```python
from build123d import *

# Parameters (mm, degrees)
SKETCH1_W           = 92.6
SKETCH1_H           = 300
BOSS_EXTRUDE1_DEPTH = 3
SKETCH3_R           = 2.25
SKETCH3_W           = 8.48
SKETCH3_H           = 51.5
SKETCH3_H_2         = 50
SKETCH3_W_2         = 5
SKETCH3_H_3         = 53
CUT_EXTRUDE2_DEPTH  = 10
FILLET1_R           = 2
SKETCH4_R           = 1.85
CUT_EXTRUDE3_DEPTH  = 5
SKETCH5_R           = 1.85
CUT_EXTRUDE4_DEPTH  = 10
SKETCH6_R           = 1.85
CUT_EXTRUDE5_DEPTH  = 8.5
CUT_EXTRUDE6_DEPTH  = 8.5
SKETCH9_R           = 1.85
CUT_EXTRUDE7_DEPTH  = 10


with BuildPart() as part:
    # Sketch1 → Boss-Extrude1 (new body)
    with BuildSketch(Plane.XY):
        Rectangle(SKETCH1_W, SKETCH1_H)
    extrude(amount=BOSS_EXTRUDE1_DEPTH)

    # Sketch3 → Cut-Extrude2 (cut)
    with BuildSketch(Plane.XY):
        with Locations((-42.06, 75)):
            Circle(SKETCH3_R)
        with Locations((42.06, 125)):
            Circle(SKETCH3_R)
        with Locations((42.06, 25)):
            Circle(SKETCH3_R)
        with Locations((42.06, -75)):
            Circle(SKETCH3_R)
        with Locations((-42.06, -25)):
            Circle(SKETCH3_R)
        with Locations((-42.06, -125)):
            Circle(SKETCH3_R)
        with Locations((-42.06, 124.25)):
            Rectangle(SKETCH3_W, SKETCH3_H)
        with Locations((42.06, 75)):
            Rectangle(SKETCH3_W, SKETCH3_H_2)
        with Locations((43.8, -25)):
            Rectangle(SKETCH3_W_2, SKETCH3_H_2)
        with Locations((-43.8, 25)):
            Rectangle(SKETCH3_W_2, SKETCH3_H_3)
        with Locations((-42.06, -75)):
            Rectangle(SKETCH3_W, SKETCH3_H_3)
        with Locations((42.06, -125)):
            Rectangle(SKETCH3_W, SKETCH3_H_2)
    extrude(amount=CUT_EXTRUDE2_DEPTH, mode=Mode.SUBTRACT)

    # Fillet1
    fillet1_edges = [part.edges().sort_by_distance(p)[0] for p in [
        (46.3, -100, 1.5),
        (37.82, -100, 1.5),
        (37.82, -150, 1.5),
        (46.3, 50, 1.5),
        (46.3, 100, 1.5),
        (37.82, 100, 1.5),
        (37.82, 50, 1.5),
        (-46.3, -48.5, 1.5),
        (-46.3, -101.5, 1.5),
        (-37.82, -101.5, 1.5),
        (-37.82, -48.5, 1.5),
        (41.3, 0, 1.5),
        (41.3, -50, 1.5),
        (46.3, -50, 1.5),
        (46.3, 0, 1.5),
        (46.3, 150, 1.5),
        (-46.3, 51.5, 1.5),
        (-46.3, -150, 1.5),
        (-46.3, -1.5, 1.5),
        (-41.3, -1.5, 1.5),
        (-41.3, 51.5, 1.5),
        (-46.3, 98.5, 1.5),
        (-37.82, 98.5, 1.5),
        (-37.82, 150, 1.5),
    ]]
    fillet(fillet1_edges, radius=FILLET1_R)

    # Sketch4 → Cut-Extrude3 (cut)
    with BuildSketch(Plane(origin=(0, 0, 0), x_dir=(-1, 0, 0), z_dir=(0, 0, -1))):
        with Locations((8.125, -47.8)):
            Circle(SKETCH4_R)
        with Locations((-8.125, -78)):
            Circle(SKETCH4_R)
    extrude(amount=-CUT_EXTRUDE3_DEPTH, mode=Mode.SUBTRACT)

    # Sketch5 → Cut-Extrude4 (cut)
    with BuildSketch(Plane(origin=(0, 0, 0), x_dir=(-1, 0, 0), z_dir=(0, 0, -1))):
        with Locations((-15, -12)):
            Circle(SKETCH5_R)
        with Locations((15, -12)):
            Circle(SKETCH5_R)
        with BuildLine():
            Line((-22.1, -18.1), (-34.1, -18.1))
            ThreePointArc((-34.1, -18.1), (-35.514213562, -17.514213562), (-36.1, -16.1))
            Line((-36.1, -16.1), (-36.1, 4.9))
            ThreePointArc((-36.1, 4.9), (-35.514213562, 6.314213562), (-34.1, 6.9))
            Line((-34.1, 6.9), (-22.1, 6.9))
            ThreePointArc((-22.1, 6.9), (-20.685786438, 6.314213562), (-20.1, 4.9))
            Line((-20.1, 4.9), (-20.1, -16.1))
            ThreePointArc((-20.1, -16.1), (-20.685786438, -17.514213562), (-22.1, -18.1))
        make_face()
        with BuildLine():
            Line((34.1, -18.1), (22.1, -18.1))
            ThreePointArc((22.1, -18.1), (20.685786438, -17.514213562), (20.1, -16.1))
            Line((20.1, -16.1), (20.1, 4.9))
            ThreePointArc((20.1, 4.9), (20.685786438, 6.314213562), (22.1, 6.9))
            Line((22.1, 6.9), (34.1, 6.9))
            ThreePointArc((34.1, 6.9), (35.514213562, 6.314213562), (36.1, 4.9))
            Line((36.1, 4.9), (36.1, -16.1))
            ThreePointArc((36.1, -16.1), (35.514213562, -17.514213562), (34.1, -18.1))
        make_face()
    extrude(amount=-CUT_EXTRUDE4_DEPTH, mode=Mode.SUBTRACT)

    # Sketch6 → Cut-Extrude5 (cut)
    with BuildSketch(Plane(origin=(0, 0, 0), x_dir=(-1, 0, 0), z_dir=(0, 0, -1))):
        with Locations((16.5, 55.5)):
            Circle(SKETCH6_R)
        with Locations((-16.5, 55.5)):
            Circle(SKETCH6_R)
        with Locations((-16.5, 75.5)):
            Circle(SKETCH6_R)
        with Locations((16.5, 75.5)):
            Circle(SKETCH6_R)
    extrude(amount=-CUT_EXTRUDE5_DEPTH, mode=Mode.SUBTRACT)

    # Sketch7 → Cut-Extrude6 (cut)
    with BuildSketch(Plane(origin=(0, 0, 0), x_dir=(-1, 0, 0), z_dir=(0, 0, -1))):
        with BuildLine():
            Line((22.5, 90), (-22.5, 90))
            ThreePointArc((-22.5, 90), (-29.571067812, 92.928932188), (-32.5, 100))
            Line((-32.5, 100), (-32.5, 125))
            ThreePointArc((-32.5, 125), (-29.571067812, 132.071067812), (-22.5, 135))
            Line((-22.5, 135), (22.5, 135))
            ThreePointArc((22.5, 135), (29.571067812, 132.071067812), (32.5, 125))
            Line((32.5, 125), (32.5, 100))
            ThreePointArc((32.5, 100), (29.571067812, 92.928932188), (22.5, 90))
        make_face()
        with BuildLine():
            Line((25, -143), (-25, -143))
            ThreePointArc((-25, -143), (-28.535533906, -141.535533906), (-30, -138))
            Line((-30, -138), (-30, -98))
            ThreePointArc((-30, -98), (-28.535533906, -94.464466094), (-25, -93))
            Line((-25, -93), (25, -93))
            ThreePointArc((25, -93), (28.535533906, -94.464466094), (30, -98))
            Line((30, -98), (30, -138))
            ThreePointArc((30, -138), (28.535533906, -141.535533906), (25, -143))
        make_face()
    extrude(amount=-CUT_EXTRUDE6_DEPTH, mode=Mode.SUBTRACT)

    # Sketch9 → Cut-Extrude7 (cut)
    with BuildSketch(Plane(origin=(0, 0, 0), x_dir=(-1, 0, 0), z_dir=(0, 0, -1))):
        with Locations((-10.5, 142.75)):
            Circle(SKETCH9_R)
        with Locations((4.5, 142.75)):
            Circle(SKETCH9_R)
    extrude(amount=-CUT_EXTRUDE7_DEPTH, mode=Mode.SUBTRACT)


solid = part.part
```
Geometry check sheet. Reference: the model listing, model coordinates, mm. A direction names the side the tool comes from. Round coordinates to 2 decimals unless told otherwise and drop trailing zeros. Order: outer loops, then holes, each group sorted by start corner. A loop starts at its lowest first (then second) coordinate and runs counter-clockwise, first axis right, second up. Notation, with made-up numbers: (0, 34.5) -> (14, 34.5) arc R21 ccw to (14, 49.5) -> close; hole circle Ø5 at (-1.5, -0.5). An arc over 180 degrees is marked (long way). Return JSON: item names as keys, results as strings. Group by question number.
Q1. Tool access check on faces 1 (the cylindrical face through (-28, -94, 1)), 2 (the flat face through (-1, 2, 0)). Record the directions out of +Z, -Z, +X, -X, +Y, -Y that give a thin tool (end or side, any length) a straight path to the whole face; none if there is none.
Q2. Section check A-A, the plane z = 0.95. Count the separate pieces of the cut face and the enclosed holes in it, plus the area to 3 significant figures.
Q3. Section check B-B, the plane y = -59.5. Record the boundary of the cut face in (x, z).
Q4. Gauge pin test, flat ends, axial feed: pin 1 (1.5 mm diameter, centred on y = -2, z = 2, fed in from +X); pin 2 (1.5 mm diameter, centred on y = -108.5, z = 2, fed in from +X). Record the tip position at first contact, or that the pin passes through.
Q5. Material ranges on probe 1 along X at (y, z) = (142.75, 1.6); probe 2 along Y at (x, z) = (-8.5, 2.8); probe 3 along Y at (x, z) = (-12.5, 2.85), recorded low to high. Write a range as from..to.
Q6. Release check for a two-part mould opening along X. For faces 3 (the cylindrical face through (29, -95, 1)), 4 (the flat face through (-1, 2, 3)) record: released by +X, released by -X, zero draft, split by the parting line, or undercut.
Numbers:
{
 "1": {"face 1": "+Z, -Z", "face 2": "-Z, +X, -X, +Y, -Y"},
 "2": {"separate pieces": "1", "enclosed holes": "20", "area": "18,700 mm^2"},
 "3": {"outline": "(-37.82, 0) -> (46.3, 0) -> (46.3, 3) -> (-37.82, 3) -> close"},
 "4": {"pin 1": "x = 41.45", "pin 2": "x = 37.82"},
 "5": {"probe 1": "-37.82..-6.35, -2.65..8.65, 12.35..46.3", "probe 2": "-150..-143, -93..-49.61, -45.99..90, 135..150", "probe 3": "-150..-143, -93..90, 135..150"},
 "6": {"face 3": "undercut", "face 4": "zero draft"}
}
